Source: CAD feature listing. Evaluate the final solid. Frame: model axes, mm. A direction names the side the tool comes from. Coordinates: 2 decimals unless noted, no trailing zeros. Write each loop counter-clockwise with the first axis right and the second up, starting at its lowest first coordinate (ties: lowest second). Pieces come first, ordered by that corner, then holes. Notation, with made-up numbers: M 34,17.25 L 89,17.25 A13 ccw 89,24.25 Z; hole C 60,-6.5 d6. An arc over 180 degrees is marked long. One line per item, written item: value. Start each with the question number.
Item 1: Cut plane C-C, the plane y = 94. Output: boundary loops of the cut face in (x, z).
Item 2: Cut plane D-D, the plane z = 43.5. Output: boundary loops of the cut face in (x, y).
Item 3: Mould query, pull axis X, two halves, no side actions, for faces 6 (the flat face through (0, -115, -63)), 7 (the flat face through (10, -34, 81)), 8 (the flat face through (-7.5, 0.5, 82.9)), 9 (the flat face through (0, -1, -55)). Classes: released by +X, released by -X, zero draft, split by the parting line, or undercut.
Item 4: Set-up query: faces 1 (the flat face through (12, -2, 1)), 2 (the flat face through (11, -110, 18)), 3 (the flat face through (0, -2, 55)), 4 (the flat face through (7, -115, -60)), 5 (the flat face through (0, 0, 80.4)). Return all of +Z, -Z, +X, -X, +Y, -Y with unobstructed straight access to the full face (end or side cutting, diameter ignored); none if empty.
Item 5: Cut plane A-A, the plane y = -19. State how many separate pieces and enclosed holes the cut face has, then the cut area to 3 significant figures.
Item 6: Pin query (flat end, axial travel): P1, Ø9, axis at x = 0, z = -57, coming from the -Y side; P2, Ø11, axis at x = 0.5, y = -113.5, coming from the +Z side; P3, Ø10, axis at y = -23, z = 73.5, coming from the +X side. Return the tip coordinate at first contact, or that it passes through.
Item 7: Ray query, L1, parallel to Y at x = -9.65, z = -59; L2, parallel to Z at x = -10.15, y = -116; L3, parallel to X at y = -102.5, z = 26. Return the intervals inside material, ascending. Write a range as from..to.
Item 8: Cut plane B-B, the plane x = -0.5. Output: boundary loops of the cut face in (y, z).
```python
from build123d import *

# Parameters (mm, degrees)
SKETCH1_W           = 240
SKETCH1_H           = 130
BOSS_EXTRUDE1_DEPTH = 12
SKETCH2_W           = 220
SKETCH2_H           = 110
CUT_EXTRUDE2_DEPTH  = 10
CUT_EXTRUDE3_DEPTH  = 137.839321834
SKETCH4_W           = 20
SKETCH4_H           = 127
BOSS_EXTRUDE2_DEPTH = 25.4
CHAMFER1_SIZE       = 25
SHELL1_START        = -10
SHELL1_DEPTH        = 20
FILLET1_R           = 5
CHAMFER2_SIZE       = 5
SKETCH6_W           = 10
SKETCH6_H           = 120
CUT_EXTRUDE5_DEPTH  = 153.145193812
SKETCH9_W           = 14
SKETCH9_H           = 8
CUT_EXTRUDE7_DEPTH  = 10
SKETCH11_R          = 0.95
CUT_EXTRUDE8_DEPTH  = 153.145193812
FILLET3_R           = 4


with BuildPart() as part:
    # Sketch1 → Boss-Extrude1 (new body)
    with BuildSketch(Plane.YZ):
        Rectangle(SKETCH1_W, SKETCH1_H)
    extrude(amount=-BOSS_EXTRUDE1_DEPTH)

    # Sketch2 → Cut-Extrude2 (cut)
    with BuildSketch(Plane.YZ):
        Rectangle(SKETCH2_W, SKETCH2_H)
    extrude(amount=-CUT_EXTRUDE2_DEPTH, mode=Mode.SUBTRACT)

    # Sketch3 → Cut-Extrude3 (cut, through all)
    with BuildSketch(Plane.YZ.offset(-10)):
        Polygon((0, 1.051462224), (-1, 0.324919696), (-0.618033989, -0.850650808), (0.618033989, -0.850650808), (1, 0.324919696), align=None)
    extrude(amount=-CUT_EXTRUDE3_DEPTH, mode=Mode.SUBTRACT)

    # Mirror6: part across plane


with BuildPart() as part_1:
    add(part.part)
    add(part.part.mirror(Plane.ZY))

    # Sketch4 → Boss-Extrude2 (add)
    with BuildSketch(Plane.XY.offset(65)):
        Rectangle(SKETCH4_W, SKETCH4_H)
    extrude(amount=BOSS_EXTRUDE2_DEPTH)

    # Chamfer1
    chamfer1_edges = [part_1.edges().sort_by_distance(p)[0] for p in [
        (0, 63.5, 90.4),
        (0, -63.5, 90.4),
    ]]
    chamfer(chamfer1_edges, length=CHAMFER1_SIZE)

    # Shell1: read off the stored shape, not the designer's step
    # Shell1 outline → Shell1 (cut)
    with BuildSketch(Plane.YZ.offset(SHELL1_START)):
        Polygon((-49.757864376, 65), (49.757864376, 65), (34.357864376, 80.4), (-34.357864376, 80.4), align=None)
    extrude(amount=SHELL1_DEPTH, mode=Mode.SUBTRACT)

    # Fillet1
    # the kernel refuses this fillet: 5 mm, written as the material it takes off along each edge
    with BuildSketch(Plane(origin=(5, -36.428932188, 85.4), x_dir=(0, 0, 1), z_dir=(1, 0, 0))) as fillet1_piece_1_section:
        Polygon((0, 0), (FILLET1_R * 1.02, 0), (FILLET1_R * 1.02, FILLET1_R * 0.422497833621), (FILLET1_R * 0.72124891681, FILLET1_R * 0.72124891681), align=None)
    fillet1_piece_1 = extrude(amount=FILLET1_R * 1.02, mode=Mode.PRIVATE)
    fillet1_piece_1 = fillet1_piece_1 - Plane(origin=(5, -36.428932188, 85.4), x_dir=(0, 0.3826834323650898, -0.9238795325112867), z_dir=(1, 0, 0)) * Sphere(FILLET1_R, mode=Mode.PRIVATE)
    add(fillet1_piece_1, mode=Mode.SUBTRACT)
    with BuildSketch(Plane(origin=(-5, -36.428932188, 85.4), x_dir=(0, -0.7071067811865476, 0.7071067811865476), z_dir=(-1, 0, 0))) as fillet1_piece_2_section:
        Polygon((0, 0), (FILLET1_R * 1.02, 0), (FILLET1_R * 1.02, FILLET1_R * 0.422497833621), (FILLET1_R * 0.72124891681, FILLET1_R * 0.72124891681), align=None)
    fillet1_piece_2 = extrude(amount=FILLET1_R * 1.02, mode=Mode.PRIVATE)
    fillet1_piece_2 = fillet1_piece_2 - Plane(origin=(-5, -36.428932188, 85.4), x_dir=(0, 0.3826834323650898, -0.9238795325112867), z_dir=(-1, 0, 0)) * Sphere(FILLET1_R, mode=Mode.PRIVATE)
    add(fillet1_piece_2, mode=Mode.SUBTRACT)
    with BuildSketch(Plane(origin=(-5, 36.428932188, 85.4), x_dir=(0, 0.7071067811865476, 0.7071067811865476), z_dir=(-1, 0, 0))) as fillet1_piece_3_section:
        Polygon((0, 0), (FILLET1_R * 1.02, 0), (FILLET1_R * 1.02, -FILLET1_R * 0.422497833621), (FILLET1_R * 0.72124891681, -FILLET1_R * 0.72124891681), align=None)
    fillet1_piece_3 = extrude(amount=FILLET1_R * 1.02, mode=Mode.PRIVATE)
    fillet1_piece_3 = fillet1_piece_3 - Plane(origin=(-5, 36.428932188, 85.4), x_dir=(0, -0.3826834323650898, -0.9238795325112867), z_dir=(-1, 0, 0)) * Sphere(FILLET1_R, mode=Mode.PRIVATE)
    add(fillet1_piece_3, mode=Mode.SUBTRACT)
    with BuildSketch(Plane(origin=(5, 36.428932188, 85.4), x_dir=(0, 0, 1), z_dir=(1, 0, 0))) as fillet1_piece_4_section:
        Polygon((0, 0), (FILLET1_R * 1.02, 0), (FILLET1_R * 1.02, -FILLET1_R * 0.422497833621), (FILLET1_R * 0.72124891681, -FILLET1_R * 0.72124891681), align=None)
    fillet1_piece_4 = extrude(amount=FILLET1_R * 1.02, mode=Mode.PRIVATE)
    fillet1_piece_4 = fillet1_piece_4 - Plane(origin=(5, 36.428932188, 85.4), x_dir=(0, -0.3826834323650898, -0.9238795325112867), z_dir=(1, 0, 0)) * Sphere(FILLET1_R, mode=Mode.PRIVATE)
    add(fillet1_piece_4, mode=Mode.SUBTRACT)
    with BuildSketch(Plane(origin=(10, -72.338834765, 56.561165235), x_dir=(-1, 0, 0), z_dir=(0, 0.7071067811865476, 0.7071067811865476))) as fillet1_piece_5_section:
        with BuildLine():
            CenterArc((FILLET1_R, -FILLET1_R), FILLET1_R, 90, 90)
            Line((0, -FILLET1_R), (0, 0))
            Line((0, 0), (FILLET1_R, 0))
        make_face()
    fillet1_piece_5 = extrude(amount=45.784271247, mode=Mode.PRIVATE)
    fillet1_piece_5 = split(fillet1_piece_5, bisect_by=Plane(origin=(10, -72.338834765, 65), z_dir=(0, 0, 1)), keep=Keep.TOP, mode=Mode.PRIVATE)
    add(fillet1_piece_5, mode=Mode.SUBTRACT)
    with BuildSketch(Plane(origin=(-13.437488438, -63.5, 65.4), x_dir=(0, 0, -1), z_dir=(1, 0, 0)), Plane(origin=(13.437488438, 63.5, 65.4), x_dir=(0, 0, -1), z_dir=(-1, 0, 0))) as fillet1_piece_6:
        with BuildLine():
            CenterArc((2.563265352, 4.50780246), FILLET1_R, 225, 19.363951138)
            Line((-0.972268554, 0.972268554), (0, 0))
            Line((0, 0), (0.4, 0))
        make_face()
    extrude(amount=26.874976876, mode=Mode.SUBTRACT)
    with BuildSketch(Plane(origin=(-10, -72.338834765, 56.561165235), x_dir=(0, 0.7071067811865476, -0.7071067811865476), z_dir=(0, 0.7071067811865476, 0.7071067811865476))) as fillet1_piece_7_section:
        with BuildLine():
            CenterArc((FILLET1_R, -FILLET1_R), FILLET1_R, 90, 90)
            Line((0, -FILLET1_R), (0, 0))
            Line((0, 0), (FILLET1_R, 0))
        make_face()
    fillet1_piece_7 = extrude(amount=45.784271247, mode=Mode.PRIVATE)
    fillet1_piece_7 = split(fillet1_piece_7, bisect_by=Plane(origin=(-10, -72.338834765, 65), z_dir=(0, 0, 1)), keep=Keep.TOP, mode=Mode.PRIVATE)
    add(fillet1_piece_7, mode=Mode.SUBTRACT)
    with BuildSketch(Plane(origin=(-5, -38.5, 90.4), x_dir=(0, -0.7071067811865476, -0.7071067811865476), z_dir=(1, 0, 0))) as fillet1_piece_8:
        with BuildLine():
            CenterArc((FILLET1_R * 0.414213562373, FILLET1_R), FILLET1_R, 225, 45)
            Line((-FILLET1_R * 0.292893218813, FILLET1_R * 0.292893218813), (0, 0))
            Line((0, 0), (FILLET1_R * 0.414213562373, 0))
        make_face()
    extrude(amount=10, mode=Mode.SUBTRACT)
    with BuildSketch(Plane(origin=(-10, 36.428932188, 90.4), x_dir=(0, 0, -1), z_dir=(0, -1, 0)), Plane(origin=(10, -36.428932188, 90.4), x_dir=(0, 0, -1), z_dir=(0, 1, 0))) as fillet1_piece_9:
        with BuildLine():
            CenterArc((FILLET1_R, FILLET1_R), FILLET1_R, 180, 90)
            Line((0, FILLET1_R), (0, 0))
            Line((0, 0), (FILLET1_R, 0))
        make_face()
    extrude(amount=72.857864376, mode=Mode.SUBTRACT)
    with BuildSketch(Plane(origin=(5, 38.5, 90.4), x_dir=(0, -1, 0), z_dir=(-1, 0, 0))) as fillet1_piece_10:
        with BuildLine():
            CenterArc((FILLET1_R * 0.414213562373, -FILLET1_R), FILLET1_R, 90, 45)
            Line((-FILLET1_R * 0.292893218813, -FILLET1_R * 0.292893218813), (0, 0))
            Line((0, 0), (FILLET1_R * 0.414213562373, 0))
        make_face()
    extrude(amount=10, mode=Mode.SUBTRACT)
    with BuildSketch(Plane(origin=(-10, 72.338834765, 56.561165235), x_dir=(0, -0.7071067811865476, -0.7071067811865476), z_dir=(0, -0.7071067811865476, 0.7071067811865476))) as fillet1_piece_11_section:
        with BuildLine():
            CenterArc((FILLET1_R, FILLET1_R), FILLET1_R, 180, 90)
            Line((0, FILLET1_R), (0, 0))
            Line((0, 0), (FILLET1_R, 0))
        make_face()
    fillet1_piece_11 = extrude(amount=45.784271247, mode=Mode.PRIVATE)
    fillet1_piece_11 = split(fillet1_piece_11, bisect_by=Plane(origin=(-10, 72.338834765, 65), z_dir=(0, 0, 1)), keep=Keep.TOP, mode=Mode.PRIVATE)
    add(fillet1_piece_11, mode=Mode.SUBTRACT)
    with BuildSketch(Plane(origin=(10, 72.338834765, 56.561165235), x_dir=(0, -0.7071067811865476, -0.7071067811865476), z_dir=(0, -0.7071067811865476, 0.7071067811865476))) as fillet1_piece_12_section:
        with BuildLine():
            CenterArc((FILLET1_R, -FILLET1_R), FILLET1_R, 90, 90)
            Line((0, -FILLET1_R), (0, 0))
            Line((0, 0), (FILLET1_R, 0))
        make_face()
    fillet1_piece_12 = extrude(amount=45.784271247, mode=Mode.PRIVATE)
    fillet1_piece_12 = split(fillet1_piece_12, bisect_by=Plane(origin=(10, 72.338834765, 65), z_dir=(0, 0, 1)), keep=Keep.TOP, mode=Mode.PRIVATE)
    add(fillet1_piece_12, mode=Mode.SUBTRACT)

    # Chamfer2
    chamfer2_edges = [part_1.edges().sort_by_distance(p)[0] for p in [
        (10, 0, 80.4),
        (-10, 0, 80.4),
    ]]
    chamfer(chamfer2_edges, length=CHAMFER2_SIZE - 0.0001)  # a hair under: the kernel refuses the full size

    # Sketch6 → Cut-Extrude5 (cut, through all)
    with BuildSketch(Plane(origin=(-12, 0, 0), x_dir=(0, -1, 0), z_dir=(-1, 0, 0))):
        with Locations((115, 5)):
            Rectangle(SKETCH6_W, SKETCH6_H)
    extrude(amount=-CUT_EXTRUDE5_DEPTH, mode=Mode.SUBTRACT)

    # Sketch9 → Cut-Extrude7 (cut)
    with BuildSketch(Plane.XZ.offset(120)):
        with Locations((0, -59)):
            Rectangle(SKETCH9_W, SKETCH9_H)
    extrude(amount=-CUT_EXTRUDE7_DEPTH, mode=Mode.SUBTRACT)

    # Sketch11 → Cut-Extrude8 (cut, through all)
    with BuildSketch(Plane(origin=(-12, 0, 0), x_dir=(0, -1, 0), z_dir=(-1, 0, 0))):
        with Locations(Location((116, -59, 0), (0, 0, 90))):
            Circle(SKETCH11_R)
    extrude(amount=-CUT_EXTRUDE8_DEPTH, mode=Mode.SUBTRACT)

    # Fillet3
    fillet3_edges = [part_1.edges().sort_by_distance(p)[0] for p in [
        (9.5, -120, -55),
        (-9.5, -120, -55),
    ]]
    fillet(fillet3_edges, radius=FILLET3_R)


solid = part_1.part
```
From the geometry:
1. outline: M -12,-65 L 12,-65 L 12,65 L -12,65 Z; hole M -10,-55 L 10,-55 L 10,55 L -10,55 Z
2. outline: M -12,-110 L -10,-110 L -10,110 L 10,110 L 10,-110 L 12,-110 L 12,120 L -12,120 Z
3. face 6: undercut
3. face 7: released by +X
3. face 8: released by -X
3. face 9: undercut
4. face 1: +Z, -Z, +X, +Y, -Y
4. face 2: +Z, +X, -X, -Y
4. face 3: -Y
4. face 4: +Z, -Y
4. face 5: +X, -X
5. separate pieces: 2
5. enclosed holes: 1
5. area: 1,080 mm²
6. P1: stops at y = -110
6. P2: stops at z = 65
6. P3: passes through
7. L1: y = -120..-116.95, -115.05..120
7. L2: z = -65..-59.95, -58.05..-55
7. L3: x = -12..-10, 10..12
8. outline: M -120,-65 L 120,-65 L 120,65 L 63.5,65 A5 ccw 62.53,66.37 L 39.96,88.94 A5 ccw 36.43,90.4 L -36.43,90.4 A5 ccw -39.96,88.94 L -62.53,66.37 A5 ccw -63.5,65 L -110,65 L -110,55 L 110,55 L 110,-55 L -110,-55 L -110,-63 L -120,-63 Z; hole M -49.76,65 L 49.76,65 L 34.36,80.4 L -34.36,80.4 Z
